```python
from build123d import *

# Parameters (mm, degrees)
SKETCH2_R           = 150
BOSS_EXTRUDE2_DEPTH = 100
SKETCH1_R           = 35
BOSS_EXTRUDE1_DEPTH = 60
FILLET1_R           = 5
CUT_EXTRUDE4_DEPTH  = 30
CIRPATTERN2_COUNT   = 4
SKETCH8_R           = 35
CUT_EXTRUDE5_DEPTH  = 266.706605172
SKETCH9_R           = 50
CUT_EXTRUDE6_DEPTH  = 30


with BuildPart() as part:
    # Sketch2 → Boss-Extrude2 (new body)
    with BuildSketch(Plane(origin=(0, 0, 0), x_dir=(0, 0, -1), z_dir=(1, 0, 0))):
        with Locations(Location((0, 0, 0), (0, 0, 180))):
            Circle(SKETCH2_R)
    extrude(amount=BOSS_EXTRUDE2_DEPTH)

    # Sketch1 → Boss-Extrude1 (add)
    with BuildSketch(Plane(origin=(100, 0, 0), x_dir=(0, 0, -1), z_dir=(1, 0, 0))):
        Circle(SKETCH1_R)
    extrude(amount=BOSS_EXTRUDE1_DEPTH)

    # Fillet1
    fillet1_edges = [part.edges().sort_by_distance(p)[0] for p in [
        (0, 0, -150),
        (100, 0, -150),
    ]]
    fillet(fillet1_edges, radius=FILLET1_R)

    # Sketch7 → Cut-Extrude4 (cut)
    with BuildSketch(Plane.ZY):
        with BuildLine():
            Line((-20, 128.452325787), (-20, 20))
            Line((-20, 20), (-128.452325787, 20))
            ThreePointArc((-128.452325787, 20), (-91.923881554, 91.923881554), (-20, 128.452325787))
        make_face()
    cut_extrude4 = extrude(amount=-CUT_EXTRUDE4_DEPTH, mode=Mode.SUBTRACT)

    # CirPattern2: Cut-Extrude4 ×4 about axis
    cirpattern2_axis = Axis((0, 0, 0), (1, 0, 0))
    for i in range(1, CIRPATTERN2_COUNT):
        add(cut_extrude4.rotate(cirpattern2_axis, i * 360 / CIRPATTERN2_COUNT), mode=Mode.SUBTRACT)

    # Sketch8 → Cut-Extrude5 (cut, through all)
    with BuildSketch(Plane(origin=(160, 0, 0), x_dir=(0, 0, -1), z_dir=(1, 0, 0))):
        Circle(SKETCH8_R)
    extrude(amount=-CUT_EXTRUDE5_DEPTH, mode=Mode.SUBTRACT)

    # Sketch9 → Cut-Extrude6 (cut)
    with BuildSketch(Plane.ZY):
        Circle(SKETCH9_R)
    extrude(amount=-CUT_EXTRUDE6_DEPTH, mode=Mode.SUBTRACT)


solid = part.part
```
Can you work these out from the model? Positions are in its coordinate system, mm. A direction names the side the tool comes from. Give positions to 0.01 mm unless a question says otherwise; leave off trailing zeros. Write each loop counter-clockwise with the first axis right and the second up, starting at its lowest first coordinate (ties: lowest second). Pieces come first, ordered by that corner, then holes. Notation, with made-up numbers: (12.25, 66) - (34.25, 66) arc R27 cw to (34.25, 105) - close; hole circle Ø6 at (65, -9.5). An arc over 180 degrees is marked (long way). Write item = value, one per line. Start each with the question number.
1. For pin 1 (9 mm diameter, centred on x = 20, z = -101, fed in from +Y); pin 2 (24 mm diameter, centred on x = 10.5, y = -89.5, fed in from -Z); pin 3 (1.5 mm diameter, centred on x = 75, z = -18.5, fed in from -Y), each with a flat end and sliding along its axis, tell me the tip position at first contact or that it passes through.
2. Please list where these lines run through material, in increasing order: line 1 (Y direction, x = 75, z = 0); line 2 (Y direction, x = 10, z = 86.5); line 3 (X direction, y = 52, z = 86).
3. Imagine slicing it at A-A (y = 0). Please give me the cut outline in (x, z), and give its area (3 significant figures).
4. Imagine slicing it at C-C (x = 17). Please give me the cut outline in (y, z).
5. Thinking about a two-plate mould opening in Z: for faces 1 (the face through (49.37, 133.076, 69.216)), 2 (the face through (15, -20, 87)), 3 (the face through (0, -54, 10)), which applies, released by +Z, released by -Z, zero draft, split by the parting line, or undercut?
6. On a 3-axis mill with a long thin cutter (end or side, diameter ignored), from which of +Z, -Z, +X, -X, +Y, -Y can I reach the whole of each face in a straight line? I mean faces 4 (the face through (65, -21, 28)), 5 (the face through (30, -27, -27)). Say none if no direction works.
7. Imagine slicing it at D-D (x = 34). Please give me the cut outline in (y, z), and give its area (3 significant figures).
Worked answers:
q1.pin_1 = 114.84
q1.pin_2 = -128.43
q1.pin_3 = -148.95
q2.line_1 = -150 to -35, 35 to 150
q2.line_2 = -122.55 to -97.05, -20 to 20, 97.05 to 122.55
q2.line_3 = 30 to 100
q3.outline = (0, -145) arc R5 ccw to (5, -150) - (95, -150) arc R5 ccw to (100, -145) - (100, -35) - (30, -35) - (30, -50) - (0, -50) - close; (0, 50) - (30, 50) - (30, 35) - (100, 35) - (100, 145) arc R5 ccw to (95, 150) - (5, 150) arc R5 ccw to (0, 145) - close
q3.area = 22,100 mm2
q4.outline = circle Ø300 at (0, 0); hole (-128.45, -20) arc R130 ccw to (-20, -128.45) - (-20, -45.83) arc R50 ccw to (20, -45.83) - (20, -128.45) arc R130 ccw to (128.45, -20) - (45.83, -20) arc R50 ccw to (45.83, 20) - (128.45, 20) arc R130 ccw to (20, 128.45) - (20, 45.83) arc R50 ccw to (-20, 45.83) - (-20, 128.45) arc R130 ccw to (-128.45, 20) - (-45.83, 20) arc R50 ccw to (-45.83, -20) - close
q5.face_1 = split by the parting line
q5.face_2 = undercut
q5.face_3 = zero draft
q6.face_4 = +X, -X
q6.face_5 = -X
q7.outline = circle Ø300 at (0, 0); hole circle Ø70 at (0, 0)
q7.area = 66,800 mm2
